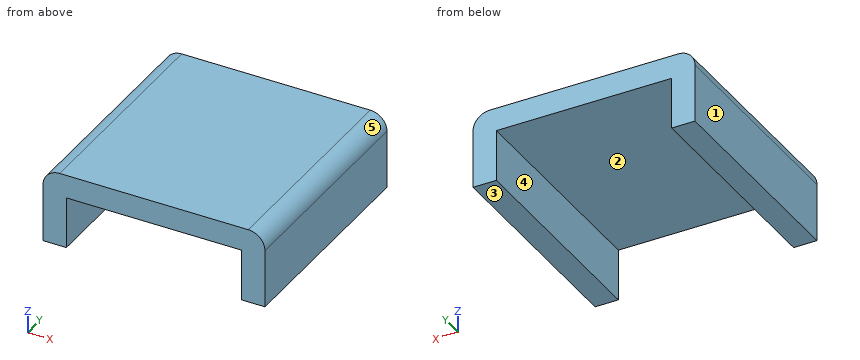
```python
from build123d import *

# Parameters (mm, degrees)
BOSS_EXTRU_1_DEPTH = 26.5
CONG_1_R           = 2


with BuildPart() as part:
    # Esquisse1 → Boss.-Extru.1 (new body)
    with BuildSketch(Plane(origin=(0, 0, 0), x_dir=(1, 0, 0), z_dir=(0, 1, 0))):
        Polygon((-13.3, 0), (13.3, 0), (13.3, 9), (10.5, 9), (10.5, 2.8), (-10.5, 2.8), (-10.5, 9), (-13.3, 9), align=None)
    extrude(amount=BOSS_EXTRU_1_DEPTH)

    # Congé1
    cong_1_edges = [part.edges().sort_by_distance(p)[0] for p in [
        (13.3, 13.25, 0),
        (-13.3, 13.25, 0),
    ]]
    fillet(cong_1_edges, radius=CONG_1_R)


solid = part.part
```
Can you work these out from the model? Positions are in its coordinate system, mm. Face numbers are marked on the shaded views. A direction names the side the tool comes from. Coordinates: 2 decimals unless noted, no trailing zeros. Loops run counter-clockwise (first coordinate to the right, second up) from the corner with the lowest first, then second, coordinate; pieces in that order, holes last.
1) Imagine slicing it at C-C on x = 7. List the corners of the cut face in (y, z) for me, plus the area to 3 significant figures.
2) Thinking about a two-plate mould opening in X: for the marked faces 3, 4 and 5, which applies, pulls with the +X half, pulls with the -X half, needs draft (parallel to the pull), parting line crosses it, or undercut?
3) Imagine slicing it at A-A on z = -5.75. List the corners of the cut face in (x, y) for me.
4) For pin 1 (6.5 mm diameter, centred on x = 2.5, y = 7, fed in from -Z), with a flat end and sliding along its axis, tell me the tip position at first contact or that it passes through.
5) Which directions (+Z, -Z, +X, -X, +Y, -Y) give clear straight access to the entire face, cutting with the end or side of a thin tool? Please do the marked faces 1 and 2.
6) Imagine slicing it at D-D on z = -0.5. List the corners of the cut face in (x, y) for me.
7) I need wall thicknesses on probe 1 along X at (y, z) = (7, -3.5); probe 2 along Z at (x, y) = (9, 21); probe 3 along Z at (x, y) = (12.25, 5.75). Which ranges of each line are inside material? Lowest first, please.
8) Imagine slicing it at B-B on y = 23. List the corners of the cut face in (x, z) for me, plus the area to 3 significant figures.
Completed:
1. outline: (0, -2.8) - (26.5, -2.8) - (26.5, 0) - (0, 0) - close
1. area: 74.2 mm2
2. face 3: needs draft
2. face 4: undercut
2. face 5: pulls with the +X half
3. outline: (-13.3, 0) - (-10.5, 0) - (-10.5, 26.5) - (-13.3, 26.5) - close; (10.5, 0) - (13.3, 0) - (13.3, 26.5) - (10.5, 26.5) - close
4. pin 1: stops at z = -2.8
5. face 1: +Z, -Z, -X, +Y, -Y
5. face 2: -Z, +Y, -Y
6. outline: (-12.62, 0) - (12.62, 0) - (12.62, 26.5) - (-12.62, 26.5) - close
7. probe 1: x = -13.3 to -10.5, 10.5 to 13.3
7. probe 2: z = -2.8 to 0
7. probe 3: z = -9 to -0.24
8. outline: (-13.3, -9) - (-10.5, -9) - (-10.5, -2.8) - (10.5, -2.8) - (10.5, -9) - (13.3, -9) - (13.3, -2) arc R2 ccw to (11.3, 0) - (-11.3, 0) arc R2 ccw to (-13.3, -2) - close
8. area: 107 mm2
